```python
from build123d import *

# Parameters (mm, degrees)
BOSS_EXTRUDE1_DEPTH        = 4
F_8_0_199_DIAMETER_HOLE6_D = 5.0546
CUT_EXTRUDE1_DEPTH         = 4


with BuildPart() as part:
    # Sketch1 → Boss-Extrude1 (new body)
    with BuildSketch(Plane(origin=(0, 0, 0), x_dir=(1, 0, 0), z_dir=(0, 1, 0))):
        with BuildLine():
            Line((-63.720091023, -12.396555886), (-66.755149614, -12.396555886))
            ThreePointArc((-66.755149614, -12.396555886), (-67.5, -2.396555886), (-66.755149614, 7.603444114))
            Line((-66.755149614, 7.603444114), (-63.720091023, 7.603444114))
            ThreePointArc((-63.720091023, 7.603444114), (0, 62.103444114), (63.720091023, 7.603444114))
            Line((63.720091023, 7.603444114), (66.755149614, 7.603444114))
            ThreePointArc((66.755149614, 7.603444114), (67.5, -2.396555886), (66.755149614, -12.396555886))
            Line((66.755149614, -12.396555886), (63.720091023, -12.396555886))
            ThreePointArc((63.720091023, -12.396555886), (0, -66.896555886), (-63.720091023, -12.396555886))
        make_face()
    extrude(amount=-BOSS_EXTRUDE1_DEPTH)

    # #8 (0.199) Diameter Hole6 (through all)
    with Locations(Plane(origin=(-32.5, -4, 52.832158391), x_dir=(0, 0, -1), z_dir=(0, -1, 0))):
        with Locations((0, 0), (0, 65), (100.871205009, 65), (100.871205009, 0)):
            Hole(F_8_0_199_DIAMETER_HOLE6_D / 2)

    # Sketch4 → Cut-Extrude1 (cut)
    with BuildSketch(Plane.XZ.offset(4)):
        Polygon((17.425968137, -23.074858179), (14.612549904, -20.505660279), (24.204222064, -10.002232211), (27.017640296, -12.571430111), align=None)
        Polygon((28.385745934, -33.083266376), (25.92935527, -30.840104068), (35.52102743, -20.336676), (37.977418094, -22.579838308), align=None)
        Polygon((-26.832584157, -1.852037702), (-30.62128677, -1.449753587), (-29.119426074, 12.694736168), (-25.330723461, 12.292452053), align=None)
        Polygon((-42.072412194, -0.233874083), (-45.380321989, 0.117359492), (-43.878461293, 14.261849248), (-40.570551498, 13.910615673), align=None)
        Polygon((1.801240517, 29.503633423), (-12.149127519, 26.727051412), (-12.892854843, 30.463757136), (1.057513193, 33.240339147), align=None)
        Polygon((-1.190357845, 44.534307106), (-15.14072588, 41.757725095), (-15.79007294, 45.020236494), (-1.839704904, 47.796818505), align=None)
    extrude(amount=-CUT_EXTRUDE1_DEPTH, mode=Mode.SUBTRACT)


solid = part.part
```
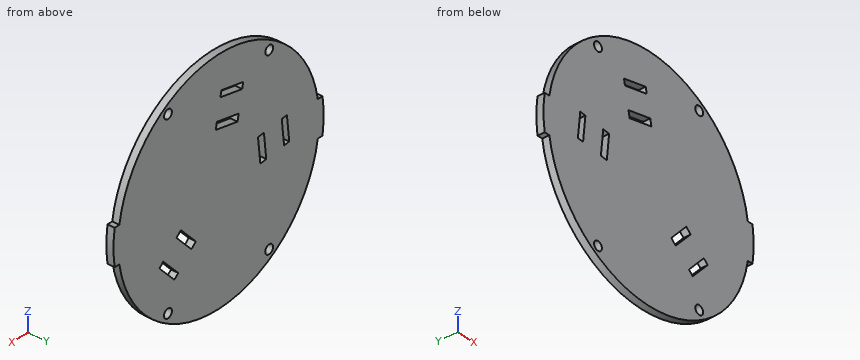
Build history of the part. All positions in model axes, mm. Give positions to 0.01 mm unless a question says otherwise; leave off trailing zeros. Loops run counter-clockwise (first coordinate to the right, second up) from the corner with the lowest first, then second, coordinate; pieces in that order, holes last. Notation, with made-up numbers: (-2, 36.25) -> (48, 36.25) arc R15 cw to (48, 47.25) -> close; hole circle Ø10 at (9, 63.5). An arc over 180 degrees is marked (long way). One line per question, with ' | ' between items. Start each with the question number.
1) Cut at A-A (x = 32.5). Give the cut face in (y, z).
2) Probe L1, parallel to X at y = -2.3, z = -26.5; L2, parallel to Z at x = 0, y = -1.4; L3, parallel to X at y = -2.8, z = 59.5. List the from-to ranges inside material, lowest first.
3) Cut at D-D (x = -32.5). Give the cut face in (y, z), plus the area to 3 significant figures.
4) Cut at B-B (z = 9). Give the cut face in (x, y).
5) Pin check, flat tips, straight feed: pin 1 (1.5 mm diameter, centred on y = -2.5, z = -34, fed in from -X); pin 2 (2 mm diameter, centred on y = -2.5, z = 17, fed in from -X); pin 3 (1.5 mm diameter, centred on x = 48, y = -1.5, fed in from +Z); pin 4 (3 mm diameter, centred on x = 32.5, z = -48.04, fed in from +Y). Stop position of each tip, or through.
6) Cut at C-C (y = -1). Count the separate pieces of the cut face and the enclosed holes in it, plus the area to 3 significant figures.
Return value:
1) outline: (-4, -53.32) -> (0, -53.32) -> (0, -50.57) -> (-4, -50.57) -> close; (-4, -45.51) -> (0, -45.51) -> (0, -28.58) -> (-4, -28.58) -> close; (-4, -23.64) -> (0, -23.64) -> (0, 50.3) -> (-4, 50.3) -> close; (-4, 55.36) -> (0, 55.36) -> (0, 58.11) -> (-4, 58.11) -> close
2) L1: -57.66 to 29.89, 34.4 to 57.66 | L2: -62.1 to 29.15, 33.03 to 66.9 | L3: -29.99 to 29.99
3) outline: (-4, -53.32) -> (0, -53.32) -> (0, -50.57) -> (-4, -50.57) -> close; (-4, -45.51) -> (0, -45.51) -> (0, 50.3) -> (-4, 50.3) -> close; (-4, 55.36) -> (0, 55.36) -> (0, 58.11) -> (-4, 58.11) -> close | area: 405 mm^2
4) outline: (-67.18, -4) -> (-44.44, -4) -> (-44.44, 0) -> (-67.18, 0) -> close; (-41.09, -4) -> (-29.51, -4) -> (-29.51, 0) -> (-41.09, 0) -> close; (-25.68, -4) -> (67.18, -4) -> (67.18, 0) -> (-25.68, 0) -> close
5) pin 1: x = -53.75 | pin 2: x = -63.05 | pin 3: z = 46.3 | pin 4: through
6) separate pieces: 1 | enclosed holes: 10 | area: 12,800 mm^2
